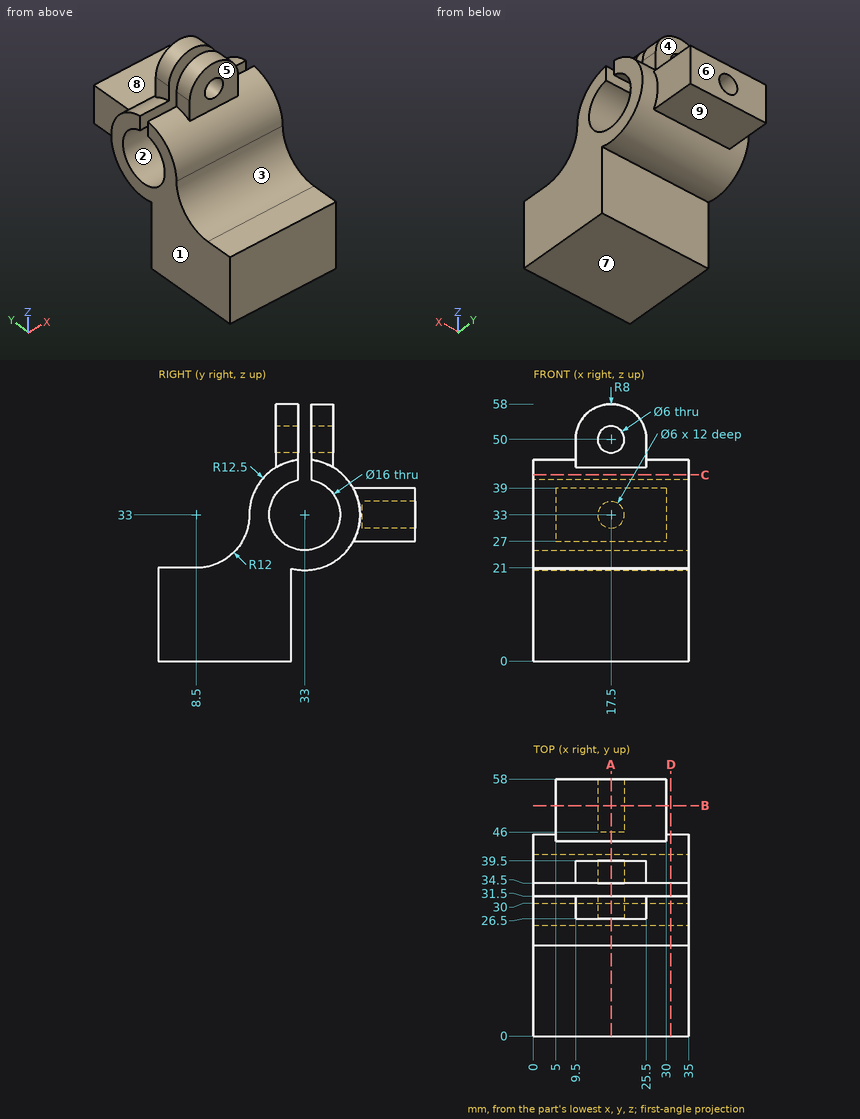
Part print with two shaded views. Sizes in mm from the minimum x, y, z corner. A direction names the side the tool comes from. Round coordinates to 2 decimals unless told otherwise and drop trailing zeros. Loops run counter-clockwise (first coordinate to the right, second up) from the corner with the lowest first, then second, coordinate; pieces in that order, holes last.
1. 3-axis set-ups, long thin cutter, end or side, ignore diameter. For the marked faces 5, 6, 7, 8 and 9: which of +Z, -Z, +X, -X, +Y, -Y reach the whole face in a straight line?
Solutions:
face 5: +Z, +X, -X, -Y
face 6: +Z, -Z, +X, -X, +Y
face 7: -Z, +X, -X, +Y, -Y
face 8: +Z, +X, -X, +Y
face 9: -Z, +X, -X, +Y
2. Slice it at D-D (x = 31). Give the cut face in (y, z).
Solutions:
outline: (0, 0) - (30, 0) - (30, 20.87) arc R12.5 ccw (long way) to (34.5, 45.41) - (34.5, 40.86) arc R8 cw (long way) to (31.5, 40.86) - (31.5, 45.41) arc R12.5 ccw to (20.5, 33) arc R12 cw to (8.5, 21) - (0, 21) - close
3. Flat gauge pins, fed straight in: pin 1 (16 mm diameter, centred on x = 14, z = 53.5, fed in from -Y); pin 2 (4.5 mm diameter, centred on x = 20.5, z = 52, fed in from +Y); pin 3 (16.5 mm diameter, centred on x = 12.5, z = 10, fed in from +Y); pin 4 (9.5 mm diameter, centred on x = 17.5, z = 33, fed in from +Y). Where does each tip first touch, or does it go through?
Solutions:
pin 1: stops at y = 26.5
pin 2: stops at y = 39.5
pin 3: stops at y = 30
pin 4: stops at y = 58
4. Slice it at A-A (x = 17.5). Count the separate pieces of the cut face and the enclosed holes in it, and give its area (3 significant figures).
Solutions:
separate pieces: 3
enclosed holes: 0
area: 1,120 mm2
5. Drill centre lines: line 1 along X through (y, z) = (36, 50); line 2 along Y through (x, z) = (12.5, 48); line 3 along X through (y, z) = (55.5, 33). Where is each one in solid material? Low to high.
Solutions:
line 1: x = 9.5 to 14.5, 20.5 to 25.5
line 2: y = 26.5 to 31.5, 34.5 to 39.5
line 3: x = 5 to 14.5, 20.5 to 30
6. Slice it at C-C (z = 42). Give the cut face in (x, y).
Solutions:
outline: (0, 24.33) - (35, 24.33) - (35, 31.5) - (0, 31.5) - close; (0, 34.5) - (35, 34.5) - (35, 41.67) - (0, 41.67) - close
7. Two-plate mould, pull along Y, no slides. Class the marked faces 1, 2, 3 and 4: pulls with the +Y half, pulls with the -Y half, needs draft (parallel to the pull), parting line crosses it, or undercut.
Solutions:
face 1: needs draft
face 2: undercut
face 3: pulls with the -Y half
face 4: pulls with the +Y half
8. Slice it at B-B (y = 52). Give the cut face in (x, z), and give its area (3 significant figures).
Solutions:
outline: (5, 27) - (30, 27) - (30, 39) - (5, 39) - close; hole circle Ø6 at (17.5, 33)
area: 272 mm2
